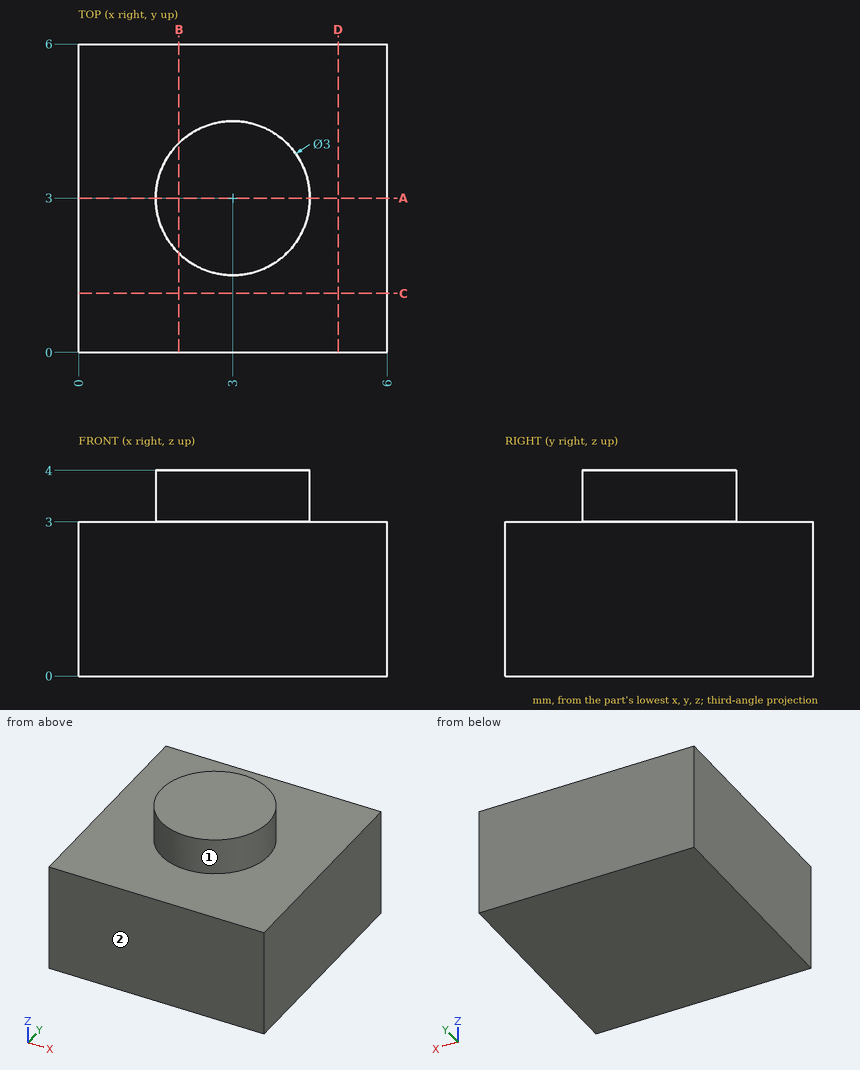
Input: dimensioned drawing with shaded views. Units: mm. Origin: part minimum x, y, z. A direction names the side the tool comes from. Give positions to 0.01 mm unless a question says otherwise; leave off trailing zeros. Loops run counter-clockwise (first coordinate to the right, second up) from the corner with the lowest first, then second, coordinate; pieces in that order, holes last. Notation, with made-up numbers: (-9, -16.5) -> (25, -16.5) arc R27 cw to (25, 19.5) -> close; hole circle Ø1 at (86.5, -32). An arc over 180 degrees is marked (long way). Use a Markdown table: item, result. Add a question column.
1) First-contact query: pin 1 (1 mm diameter, centred on x = 5, y = 3.5, fed in from +Z). Flat tip, straight axial feed; report the tip coordinate or a pass-through.
2) Section query B-B, the plane x = 1.95. Return the cut outline in (y, z), then the cut area to 3 significant figures.
3) Section query C-C, the plane y = 1.15. Return the cut outline in (x, z).
4) Section query A-A, the plane y = 3. Return the cut outline in (x, z).
5) Reachability of the marked faces 1 and 2 from +Z, -Z, +X, -X, +Y, -Y: full face, straight path, thin tool, end or side. Return the list, or none.
6) Line query: line 1 along Y through (x, z) = (3, 3.25); line 2 along Z through (x, y) = (4.2, 5.3); line 3 along X through (y, z) = (3.25, 3.45). Output: solid intervals per line, ascending. Write a range as [from, to].
Numbers:
| question | item | result |
|---|---|---|
| 1 | pin 1 | stops at z = 3 |
| 2 | outline | (0, 0) -> (6, 0) -> (6, 3) -> (4.07, 3) -> (4.07, 4) -> (1.93, 4) -> (1.93, 3) -> (0, 3) -> close |
| 2 | area | 20.1 mm2 |
| 3 | outline | (0, 0) -> (6, 0) -> (6, 3) -> (0, 3) -> close |
| 4 | outline | (0, 0) -> (6, 0) -> (6, 3) -> (4.5, 3) -> (4.5, 4) -> (1.5, 4) -> (1.5, 3) -> (0, 3) -> close |
| 5 | face 1 | +Z |
| 5 | face 2 | +Z, -Z, +X, -X, -Y |
| 6 | line 1 | y = [1.5, 4.5] |
| 6 | line 2 | z = [0, 3] |
| 6 | line 3 | x = [1.52, 4.48] |
